For this review, take the finished solid that the model builds, in its own axes (mm). Face numbers are marked on the shaded views. A direction names the side the tool comes from. Coordinates: 2 decimals unless noted, no trailing zeros. Write each loop counter-clockwise with the first axis right and the second up, starting at its lowest first coordinate (ties: lowest second). Pieces come first, ordered by that corner, then holes.
Autodesk Inventor part; units mm, degrees
ref_plane "YZ Plane" through (0, 0, 0) normal (1, 0, 0) x (0, 1, 0)
ref_plane "XZ Plane" through (0, 0, 0) normal (0, 1, 0) x (-1, 0, 0)
ref_plane "XY Plane" through (0, 0, 0) normal (0, 0, 1) x (1, 0, 0)
sketch "Sketch1" plane through (0, 0, 0) normal (0, 1, 0) x (-1, 0, 0)
  line L0 (0, 0) -> (58, 0) construction
  line L1 (58, 0) -> (58, -48) construction
  line L2 (58, -48) -> (0, -48) construction
  line L3 (0, -48) -> (0, 0) construction
  circle A0 centre (50.5, -7.5) radius 2.35
  circle A1 centre (50.5, -40.5) radius 2.35
  circle A2 centre (7.5, -7.5) radius 2.35
  circle A3 centre (7.5, -40.5) radius 2.35
  circle A4 centre (50.5, -7.5) radius 5
  circle A5 centre (50.5, -40.5) radius 5
  circle A6 centre (7.5, -7.5) radius 5
  circle A7 centre (7.5, -40.5) radius 5
  dimension "d0" = 58
  dimension "d1" = 48
  dimension "d2" = 4.7
  dimension "d3" = 4.7
  dimension "d4" = 4.7
  dimension "d5" = 4.7
  dimension "d6" = 33
  dimension "d7" = 43
  dimension "d8" = 7.5
  dimension "d9" = 7.5
  dimension "d10" = 7.5
  dimension "d11" = 7.5
  dimension "d12" = 7.5
  dimension "d13" = 7.5
  dimension "d14" = 10
  dimension "d15" = 10
  dimension "d16" = 10
  dimension "d17" = 10
extrude "Extrusion1" add sketch "Sketch1" along normal blind 12
sketch "Sketch2" plane through (-50.5, 12, -7.5) normal (0, 1, 0) x (1, 0, 0)
  line L0 (-31, -58.5) -> (74, -58.5)
  line L1 (74, -58.5) -> (74, 91.5)
  line L2 (74, 91.5) -> (-31, 91.5)
  line L3 (-31, 91.5) -> (-31, -58.5)
  circle A0 centre (0, 0) radius 2.35
  circle A1 centre (0, 33) radius 2.35
  circle A2 centre (43, 33) radius 2.35
  circle A3 centre (43, 0) radius 2.35
  circle A4 centre (43, 0) radius 2.35
  point P0 (50.5, -7.5)
  dimension "d20" = 105
  dimension "d21" = 150
  dimension "d22" = 58.5
  dimension "d23" = 31
extrude "Extrusion3" add sketch "Sketch2" along normal blind 4
sketch "Sketch3" plane through (-50.5, 16, -7.5) normal (0, 1, 0) x (1, 0, 0)
  line L0 (-31, 91.5) -> (-31, -58.5)
  line L1 (-31, -58.5) -> (-31, -38.5)
  line L2 (-31, -38.5) -> (-28, -38.5)
  line L3 (-28, -38.5) -> (-28, -55.5)
  line L4 (-28, -55.5) -> (-11, -55.5)
  line L5 (-11, -58.5) -> (-31, -58.5)
  line L6 (-28, 88.5) -> (-11, 88.5)
  line L7 (74, -58.5) -> (74, 91.5)
  line L8 (74, 91.5) -> (54, 91.5)
  line L9 (71, 71.5) -> (74, 71.5)
  line L10 (74, 71.5) -> (74, 91.5)
  line L11 (74, -58.5) -> (74, -38.5)
  line L12 (74, -38.5) -> (71, -38.5)
  line L13 (71, -38.5) -> (71, -55.5)
  line L14 (71, -55.5) -> (54, -55.5)
  line L15 (54, -58.5) -> (74, -58.5)
  line L16 (74, 91.5) -> (-31, 91.5)
  line L17 (54, 88.5) -> (71, 88.5)
  line L18 (71, 88.5) -> (71, 71.5)
  line L19 (-11, 91.5) -> (-31, 91.5)
  line L20 (-31, 91.5) -> (-31, 71.5)
  line L21 (-31, 71.5) -> (-28, 71.5)
  line L22 (-28, 71.5) -> (-28, 88.5)
  line L23 (-11, -55.5) -> (54, -55.5)
  line L24 (54, -58.5) -> (-11, -58.5)
  line L25 (-11, 91.5) -> (54, 91.5)
  line L26 (54, 88.5) -> (-11, 88.5)
  point P0 (50.5, -7.5)
  dimension "d28" = 20
  dimension "d48" = 20
  dimension "d49" = 3
  dimension "d50" = 3
  dimension "d51" = 3
  dimension "d52" = 3
  dimension "d53" = 20
  dimension "d55" = 20
  dimension "d56" = 20
  dimension "d57" = 3
  dimension "d69" = 20
  dimension "d95" = 17
  dimension "d96" = 65
  dimension "d102" = 3
  dimension "d103" = 17
  dimension "d104" = 65
  dimension "d105" = 17
extrude "Extrusion4" add sketch "Sketch3" along normal blind 28 contours L16 L8 L7 L9 L18 L17 L26 L6 L22 L21 L0 | L2 L3 L4 L23 L14 L13 L12 L7 L15 L24 L5 L0
sketch "Sketch4" plane through (-81.5, 12, 51) normal (0, 0, 1) x (1, 0, 0)
  line L0 (0, 0) -> (0, 32)
  line L1 (0, 0) -> (100, 0)
  line L2 (100, 0) -> (100, -15)
  line L3 (100, -15) -> (0, -15)
  line L4 (0, -15) -> (0, 0)
  point P0 (81.5, -12)
  dimension "d59" = 100
  dimension "d60" = 15
extrude "remove legs" cut sketch "Sketch4" against normal through all
sketch "Sketch5" plane through (-50.5, 12, -7.5) normal (0, -1, 0) x (1, 0, 0)
  circle A0 centre (0, 0) radius 2.35
  circle A1 centre (0, 0) radius 4.1
  circle A2 centre (43, 0) radius 2.35
  circle A3 centre (43, 0) radius 4.1
  circle A4 centre (43, -33) radius 2.35
  circle A5 centre (43, -33) radius 4.1
  circle A6 centre (0, -33) radius 2.35
  circle A7 centre (0, -33) radius 4.1
  circle A8 centre (0, 0) radius 2.35
  circle A9 centre (43, 0) radius 2.35
  circle A10 centre (43, -33) radius 2.35
  circle A11 centre (0, -33) radius 2.35
  point P0 (50.5, 7.5)
  dimension "d63" = 8.2
  dimension "d64" = 8.2
  dimension "d65" = 8.2
  dimension "d66" = 8.2
extrude "Extrusion6" cut sketch "Sketch5" against normal blind 4
sketch "Sketch6" plane through (-50.5, 16, -7.5) normal (0, 1, 0) x (1, 0, 0)
  line L0 (9, -17.5) -> (34, -17.5)
  line L1 (34, -17.5) -> (34, -32.5)
  line L2 (34, -32.5) -> (9, -32.5)
  line L3 (9, -32.5) -> (9, -17.5)
  line L4 (30.5, 55) -> (45.5, 55)
  line L5 (45.5, 55) -> (45.5, 80)
  line L6 (45.5, 80) -> (30.5, 80)
  line L7 (30.5, 80) -> (30.5, 55)
  circle A0 centre (43, 33) radius 4.1 construction
  circle A1 centre (0, 33) radius 4.1 construction
  circle A2 centre (0, 0) radius 4.1 construction
  circle A3 centre (43, 0) radius 4.1 construction
  point P0 (50.5, -7.5)
  dimension "d72" = 25
  dimension "d73" = 15
  dimension "d74" = 15
  dimension "d75" = 25
  dimension "d76" = 22
  dimension "d77" = 2.5
  dimension "d78" = 9
  dimension "d79" = 17.5
extrude "Extrusion7" cut sketch "Sketch6" against normal blind 10
chamfer "Chamfer1" distance 1 angle 45 4 edges at (-11.6, 12, -7.5) (-11.6, 12, -40.5) (-54.6, 12, -40.5) (-54.6, 12, -7.5)
sketch "Sketch7" plane through (-50.5, 16, -7.5) normal (0, 1, 0) x (1, 0, 0)
  line L0 (74, -38.5) -> (74, 71.5)
  line L1 (74, 42) -> (71, 42)
  line L2 (71, 42) -> (71, -9)
  line L3 (71, -9) -> (74, -9)
  line L4 (74, -9) -> (74, 42)
  line L5 (-31, 71.5) -> (-31, -38.5)
  line L6 (-31, 42) -> (-28, 42)
  line L7 (-28, 42) -> (-28, -9)
  line L8 (-28, -9) -> (-31, -9)
  line L9 (-31, -9) -> (-31, 42)
  line L10 (-31, -58.5) -> (74, -58.5)
  point P0 (50.5, -7.5)
  point P1 (74, -28.5)
  point P2 (74, 61.5)
  point P3 (-31, 67.5)
  point P4 (-31, -28.5)
  point P5 (72.5, 42)
  point P6 (-29.5, 42)
  point P7 (-31, -9)
  point P8 (74, -48.5)
  point P9 (-31, -48.5)
  dimension "d88" = 3
  dimension "d89" = 51
  dimension "d91" = 3
  dimension "d92" = 51
  dimension "d116" = 49.5
sketch "Sketch8" plane through (23.5, 12, 51) normal (1, 0, 0) x (0, 0, -1)
  circle A0 centre (61.5, 20) radius 8.5
  circle A1 centre (88.5, 20) radius 8.5
  line L0 (0, 0) -> (150, 0)
  line L1 (0, 0) -> (0, 32)
  point P0 (51, -12)
  dimension "d106" = 17
  dimension "d107" = 17
  dimension "d108" = 27
  dimension "d109" = 20
  dimension "d119" = 61.5
sketch "Sketch9" plane through (-81.5, 12, 51) normal (0, 0, 1) x (1, 0, 0)
  circle A0 centre (39, 20) radius 8.5
  circle A1 centre (66, 20) radius 8.5
  line L0 (0, 0) -> (105, 0)
  line L1 (0, 0) -> (0, 32)
  point P0 (81.5, -12)
  dimension "d113" = 17
  dimension "d114" = 17
  dimension "d115" = 20
  dimension "d124" = 20
  dimension "d125" = 39
  dimension "d126" = 27
extrude "Extrusion10" add sketch "Sketch7" along normal blind 28
extrude "Extrusion11" cut sketch "Sketch8" against normal through all
extrude "Extrusion12" cut sketch "Sketch9" against normal through all
sketch "Sketch11" plane through (-81.5, 12, -99) normal (-1, 0, 0) x (0, 0, 1)
  line L0 (20, 32) -> (3, 32)
  line L1 (3, 4) -> (20, 4)
  line L2 (20, 32) -> (7, 32)
  line L3 (7, 32) -> (7, 4)
  line L4 (7, 4) -> (20, 4)
  line L5 (20, 4) -> (20, 32)
  point P0 (99, -12)
  point P1 (20, 4)
  point P2 (7, 32)
  dimension "d127" = 13
extrude "Extrusion13" cut sketch "Sketch11" against normal through all
fillet "Fillet3" radius 4 2 edges at (20.5, 16, -24) (-78.5, 16, -24)
fillet "Fillet4" radius 4 2 edges at (-29, 16, -96) (-29, 16, 48)
sketch "Sketch12" plane through (-81.5, 12, -99) normal (-1, 0, 0) x (0, 0, 1)
  line L0 (100.5, 4) -> (130, 4)
  line L1 (130, 32) -> (150, 32)
  line L2 (130, 4) -> (143, 4)
  line L3 (143, 4) -> (143, 32)
  line L4 (143, 32) -> (130, 32)
  line L5 (130, 32) -> (130, 4)
  point P0 (99, -12)
  point P1 (130, 18)
  dimension "d132" = 13
extrude "Extrusion14" cut sketch "Sketch12" against normal through all
properties part number "TestingPlatform_base01"
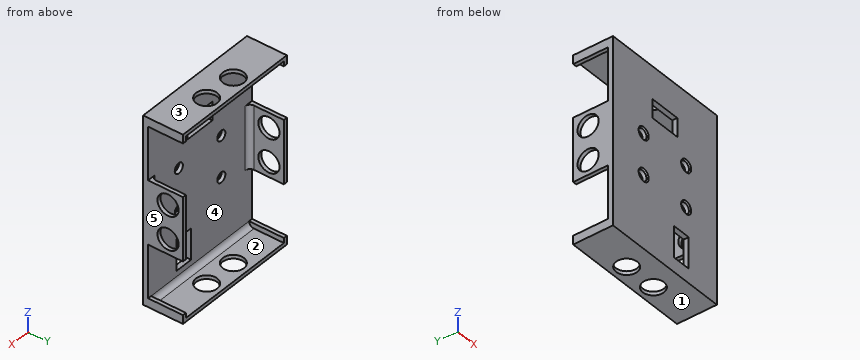
1) The part is to be moulded in two halves that separate along X. For the marked faces 3, 4 and 5, say which applies: pulls with the +X half, pulls with the -X half, needs draft (parallel to the pull), parting line crosses it, or undercut.
2) Consider section B-B (z = -27.5). Give the boundary of the cut face in (x, y).
3) For L1, parallel to X at y = 20, z = -28; L2, parallel to Z at x = -76, y = 26; L3, parallel to Y at x = -15.5, z = -98.4, list the stretches that pass through material, from the lowest coordinate up.
4) Tool access review of the marked faces 1 and 2: name each direction out of +Z, -Z, +X, -X, +Y, -Y from which nothing blocks a thin tool from reaching the whole face with its end or side.
5) Consider section A-A (x = -70). Give the boundary of the cut face in (y, z).
6) Clearance check with flat-ended pins moving along their axes: P1, Ø2, axis at x = 12, z = -14.5, coming from the +Y side; P2, Ø4, axis at x = -17, y = 37.5, coming from the -Z side. State where each tip first meets the part, or that it passes through.
7) Consider section C-C (z = -7.5). Count the separate pieces of the cut face and the enclosed holes in it, then the cut area to 3 significant figures.
Results:
1. face 3: needs draft
1. face 4: undercut
1. face 5: pulls with the +X half
2. outline: (-81.5, 12) - (23.5, 12) - (23.5, 44) - (20.5, 44) - (20.5, 20) arc R4 cw to (16.5, 16) - (-74.5, 16) arc R4 cw to (-78.5, 20) - (-78.5, 44) - (-81.5, 44) - close
3. L1: x = -81.5 to -78.5, 20.5 to 23.5
3. L2: z = -99 to -96, 48 to 51
3. L3: y = 12 to 23.5, 40.5 to 44
4. face 1: -Z, +X, -X, +Y, -Y
4. face 2: +Y
5. outline: (12, -99) - (44, -99) - (44, -96) - (20, -96) arc R4 cw to (16, -92) - (16, 44) arc R4 cw to (20, 48) - (44, 48) - (44, 51) - (12, 51) - close
6. P1: stops at y = 16
6. P2: passes through
7. separate pieces: 5
7. enclosed holes: 0
7. area: 432 mm2
